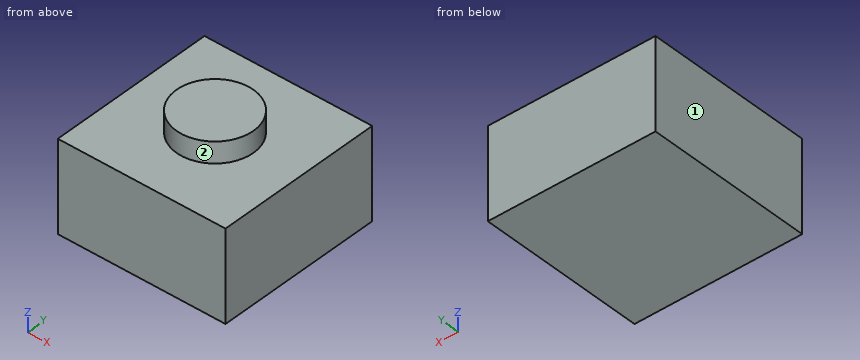
```python
from build123d import *

# Parameters (mm, degrees)
BOX010_W          = 12
BOX010_H          = 12
BOX010_DEPTH      = 6.5
CYLINDER004_R     = 2.75
CYLINDER004_DEPTH = 2.5


with BuildPart() as obj1:
    # Box010 → Box010 (new body)
    with BuildSketch(Plane.XY):
        with Locations((6, 6)):
            Rectangle(BOX010_W, BOX010_H)
    extrude(amount=BOX010_DEPTH)


with BuildPart() as obj2:
    # Cylinder004 → Cylinder004 (new body)
    with BuildSketch(Plane(origin=(6, 6, 5.5), x_dir=(1, 0, 0), z_dir=(0, 0, 1))):
        Circle(CYLINDER004_R)
    extrude(amount=CYLINDER004_DEPTH)

    # Fusion002: union obj1
    add(obj1.part)


with BuildPart() as obj2_1:
    # Fusion002 placement: moved
    add(obj2.part.moved(Location((3.5, 92, 1.1))))


solid = obj2_1.part
```
Here's how the part is built. I have some questions about the finished solid (model axes, mm). Face numbers are marked on the shaded views. A direction names the side the tool comes from. Give positions to 0.01 mm unless a question says otherwise; leave off trailing zeros. Loops run counter-clockwise (first coordinate to the right, second up) from the corner with the lowest first, then second, coordinate; pieces in that order, holes last. Notation, with made-up numbers: M -35,45.5 L -22,45.5 A18 cw -22,74.5 Z; hole C 27,-32.75 d4. An arc over 180 degrees is marked long. Put each result on its own line as item: value. Start each with the question number.
(1) For the marked faces 1 and 2, which set-ups out of +Z, -Z, +X, -X, +Y, -Y let a thin tool reach every point of the face, with its end or its side?
(2) I want a section at D-D on x = 13.75. Please give me the cut outline in (y, z), then the cut area to 3 significant figures.
(3) I want a section at C-C on y = 93.75. Please give me the cut outline in (x, z).
(4) I need wall thicknesses on line 1 along Z through (x, y) = (13.25, 96.5); line 2 along Y through (x, z) = (8, 8); line 3 along X through (y, z) = (97.5, 8.75). Which ranges of each line are inside material? Lowest first, please. Write a range as [from, to].
(5) I want a section at A-A on y = 98. Please give me the cut outline in (x, z).
(6) I want a section at B-B on x = 9.5. Please give me the cut outline in (y, z), then the cut area to 4 significant figures.
Answer block:
1. face 1: +Z, -Z, -X, +Y, -Y
1. face 2: +Z
2. outline: M 92,1.1 L 104,1.1 L 104,7.6 L 92,7.6 Z
2. area: 78.0 mm^2
3. outline: M 3.5,1.1 L 15.5,1.1 L 15.5,7.6 L 3.5,7.6 Z
4. line 1: [1.1, 7.6]
4. line 2: [95.7, 100.3]
4. line 3: [6.8, 12.2]
5. outline: M 3.5,1.1 L 15.5,1.1 L 15.5,7.6 L 12.25,7.6 L 12.25,9.1 L 6.75,9.1 L 6.75,7.6 L 3.5,7.6 Z
6. outline: M 92,1.1 L 104,1.1 L 104,7.6 L 100.75,7.6 L 100.75,9.1 L 95.25,9.1 L 95.25,7.6 L 92,7.6 Z
6. area: 86.25 mm^2
